Design review of the part shown in the three views and the two pictorial views. Dimensions are in mm from the part's minimum x, y and z. A direction names the side the tool comes from. Round coordinates to 2 decimals unless told otherwise and drop trailing zeros. Order: outer loops, then holes, each group sorted by start corner. A loop starts at its lowest first (then second) coordinate and runs counter-clockwise, first axis right, second up. Notation, with made-up numbers: M 27,0.25 L 64,0.25 A31 ccw 64,31.25 Z; hole C 36.25,-36.75 d8. An arc over 180 degrees is marked long. Use a Markdown table: item, result. Add a question column.
(1) Take a section at C-C (y = 2). Write out the cut boundary in (x, z).
(2) Take a section at A-A (x = 7.5). Write out the cut boundary in (y, z), then the cut area to 3 significant figures.
(3) To check wall thickness, follow probe 1 along Y at (x, z) = (7.5, 3.8); probe 2 along Z at (x, y) = (21.25, 10); probe 3 along Z at (x, y) = (11.25, 16.25). State the ranges of each line that lie inside material, in increasing order. Write a range as from..to.
(4) Take a section at B-B (z = 20.25). Write out the cut boundary in (x, y), then the cut area to 3 significant figures.
(5) Machinability: for the marked faces 4 and 5, which of the approach directions +Z, -Z, +X, -X, +Y, -Y give a long, thin tool a straight path to every point of the face, cutting with its end or side? Answer none if there is none.
(6) For pin 1 (1.5 mm diameter, centred on x = 4.5, y = 6.5, fed in from +Z); pin 2 (5 mm diameter, centred on x = 7.5, y = 10, fed in from +Z); pin 3 (5 mm diameter, centred on x = 24, y = 7.5, fed in from +Z); pin 4 (6 mm diameter, centred on y = 15.5, z = 17.5, fed in from -X), all flat-tipped, find the tip position at first contact; note any pin that passes through.
(7) Take a section at D-D (y = 8.5). Write out the cut boundary in (x, z).
(8) The part is to be moulded in two halves that separate along Y. For the marked faces 1, 2 and 3, say which applies: released by +Y, released by -Y, zero draft, split by the parting line, or undercut.
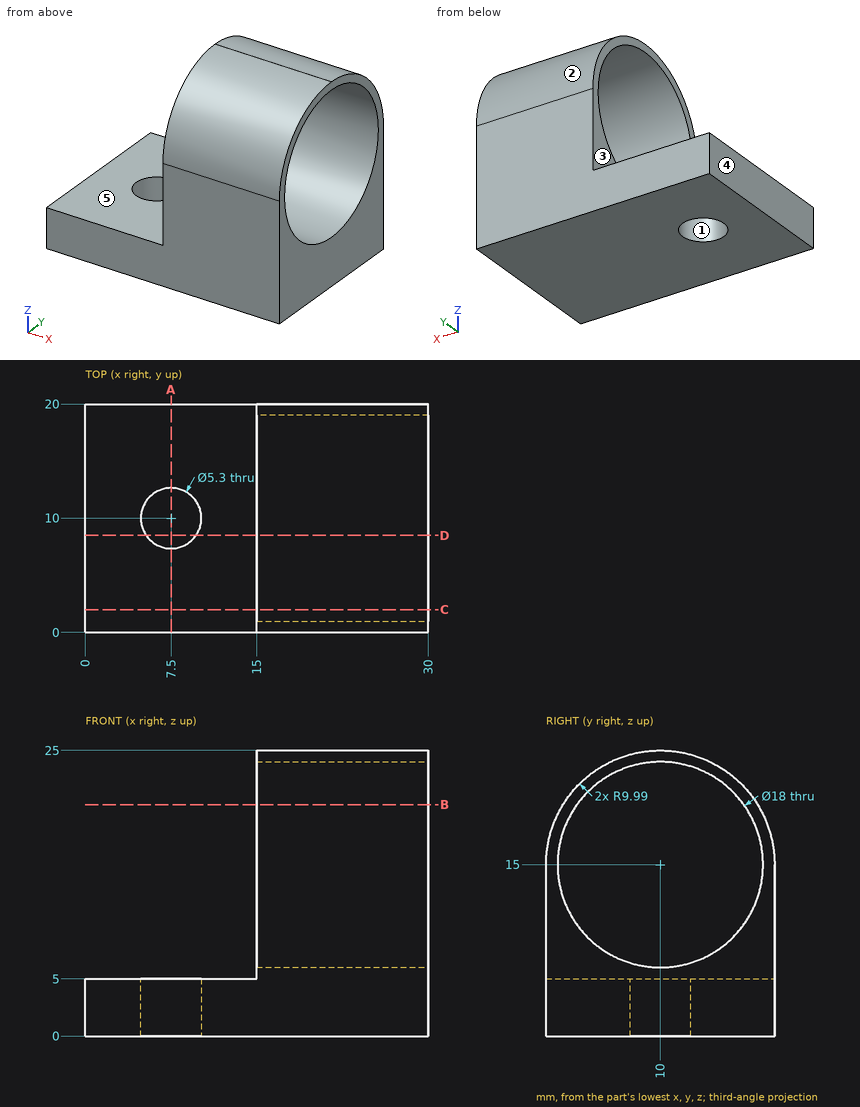
Verdict:
| question | item | result |
|---|---|---|
| 1 | outline | M 0,0 L 30,0 L 30,10.88 L 15,10.88 L 15,5 L 0,5 Z; M 15,19.12 L 30,19.12 L 30,21.01 L 15,21.01 Z |
| 2 | outline | M 0,0 L 7.35,0 L 7.35,5 L 0,5 Z; M 12.65,0 L 20,0 L 20,5 L 12.65,5 Z |
| 2 | area | 73.5 mm^2 |
| 3 | probe 1 | y = 0..7.35, 12.65..20 |
| 3 | probe 2 | z = 0..6, 24..25 |
| 3 | probe 3 | z = 0..5 |
| 4 | outline | M 15,1.48 L 30,1.48 L 30,2.69 L 15,2.69 Z; M 15,17.31 L 30,17.31 L 30,18.52 L 15,18.52 Z |
| 4 | area | 36.2 mm^2 |
| 5 | face 4 | +Z, -Z, -X, +Y, -Y |
| 5 | face 5 | +Z, -X, +Y, -Y |
| 6 | pin 1 | stops at z = 5 |
| 6 | pin 2 | passes through |
| 6 | pin 3 | stops at z = 25 |
| 6 | pin 4 | stops at x = 15 |
| 7 | outline | M 0,0 L 5.32,0 L 5.32,5 L 0,5 Z; M 9.68,0 L 30,0 L 30,6.13 L 15,6.13 L 15,5 L 9.68,5 Z; M 15,23.87 L 30,23.87 L 30,24.89 L 15,24.89 Z |
| 8 | face 1 | undercut |
| 8 | face 2 | released by +Y |
| 8 | face 3 | zero draft |
